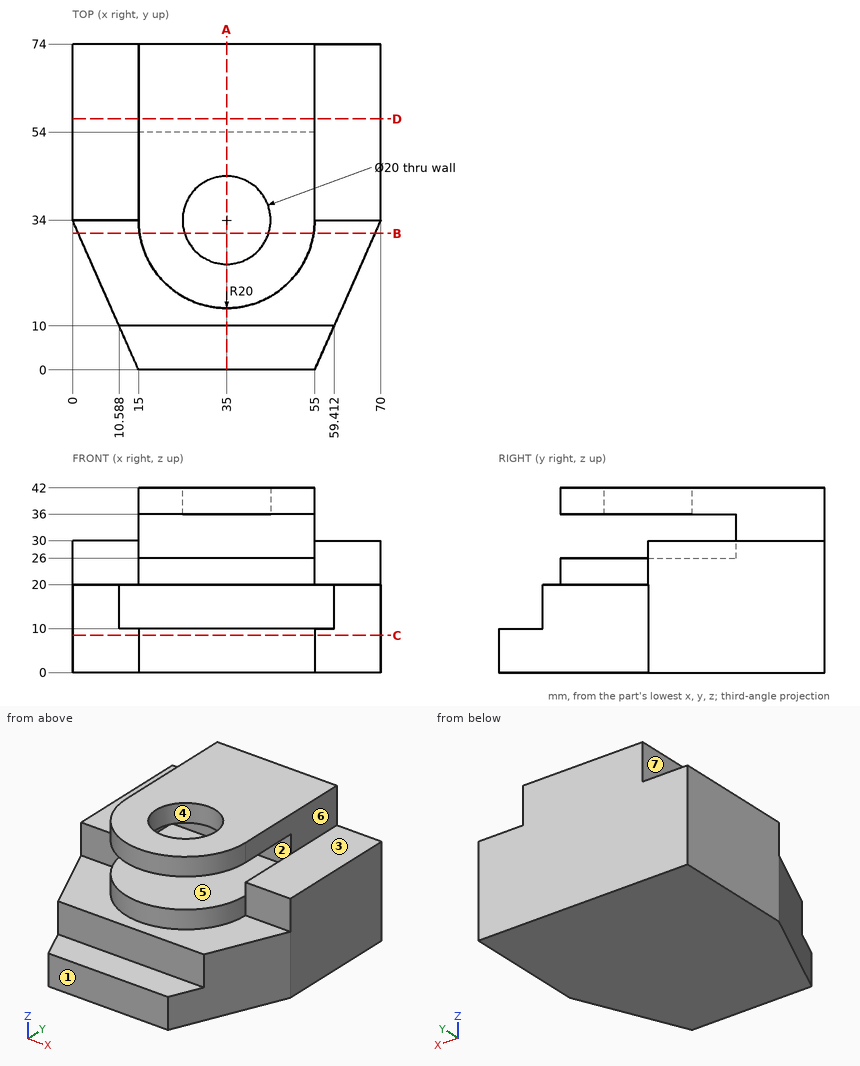
Geometry: see drawing. Coordinates: mm, zero at the bounding-box minimum. A direction names the side the tool comes from. Give positions to 0.01 mm unless a question says otherwise; leave off trailing zeros. Order: outer loops, then holes, each group sorted by start corner. A loop starts at its lowest first (then second) coordinate and runs counter-clockwise, first axis right, second up.
Q1. Section B-B on y = 31. Output: boundary loops of the cut face in (x, z).
Checked values:
outline: (1.32, 0) - (68.68, 0) - (68.68, 20) - (54.77, 20) - (54.77, 26) - (15.23, 26) - (15.23, 20) - (1.32, 20) - close; (15.23, 36) - (25.46, 36) - (25.46, 42) - (15.23, 42) - close; (44.54, 36) - (54.77, 36) - (54.77, 42) - (44.54, 42) - close
Q2. Draft query along Z for the marked faces 1, 2 and 3. Return one class per face: +Z half, -Z half, draft (parallel to the pull), parting line (faces both ways), or undercut.
Checked values:
face 1: draft
face 2: undercut
face 3: +Z half
Q3. Ray query, probe 1 along Z at (x, y) = (51, 48.5); probe 2 along Y at (x, z) = (35, 39.25); probe 3 along Z at (x, y) = (21.5, 16). Return the intervals inside material, ascending.
Checked values:
probe 1: z = 0 to 26, 36 to 42
probe 2: y = 14 to 24, 44 to 74
probe 3: z = 0 to 20
Q4. Section D-D on y = 57. Output: boundary loops of the cut face in (x, z).
Checked values:
outline: (0, 0) - (70, 0) - (70, 30) - (55, 30) - (55, 42) - (15, 42) - (15, 30) - (0, 30) - close
Q5. Section A-A on x = 35. Output: boundary loops of the cut face in (y, z), and give its area (3 significant figures).
Checked values:
outline: (0, 0) - (74, 0) - (74, 42) - (44, 42) - (44, 36) - (54, 36) - (54, 26) - (14, 26) - (14, 20) - (10, 20) - (10, 10) - (0, 10) - close; (14, 36) - (24, 36) - (24, 42) - (14, 42) - close
area: 2,180 mm2
Q6. Contact query for flat-ended pins moving along their axis: pin 1 Ø5 at (x, z) = (10, 26.5) entering from -Y; pin 2 Ø3 at (x, z) = (35.5, 16.5) entering from -Y; pin 3 Ø16.5 at (x, y) = (5, 60) entering from +Z. Output: stop coordinate, or through.
Checked values:
pin 1: stops at y = 34
pin 2: stops at y = 10
pin 3: stops at z = 30
Q7. Section C-C on z = 8.5. Output: boundary loops of the cut face in (x, y), and give its area (3 significant figures).
Checked values:
outline: (0, 34) - (15, 0) - (55, 0) - (70, 34) - (70, 74) - (0, 74) - close
area: 4,670 mm2
Q8. Set-up query: the marked faces 4, 5, 6 and 7. Return all of +Z, -Z, +X, -X, +Y, -Y with unobstructed straight access to the full face (end or side cutting, diameter ignored); none if empty.
Checked values:
face 4: +Z
face 5: -Y
face 6: +Z, +X, +Y, -Y
face 7: +Z, -X, +Y, -Y
